For this review, take the finished solid that the model builds, in its own axes (mm). A direction names the side the tool comes from. Coordinates: 2 decimals unless noted, no trailing zeros. Order: outer loops, then holes, each group sorted by start corner. A loop starts at its lowest first (then second) coordinate and runs counter-clockwise, first axis right, second up. Notation, with made-up numbers: (35.5, 64.25) -> (74.5, 64.25) arc R26 ccw to (74.5, 83.25) -> close; hole circle Ø9 at (-32, -29.75). An arc over 180 degrees is marked (long way). Write item = value, one per line. Start each with the question number.
1) Draft analysis for pull direction Y (two halves, no side actions). For faces 5 (the face through (15.266, 67.285, 4.93)), 6 (the face through (0, 19, 0)), 7 (the face through (0, 10, 18)), state which applies: +Y half, -Y half, draft (parallel to the pull), parting line (faces both ways), or undercut.
2) Machinability: for faces 1 (the face through (-21, 41, 5)), 2 (the face through (22.4, 7.5, 18.2)), 3 (the face through (0, 0, 20)), 4 (the face through (0, 34, 10)), which of the approach directions +Z, -Z, +X, -X, +Y, -Y give a long, thin tool a straight path to every point of the face, cutting with its end or side? Answer none if there is none.
3) Insertion check: pin 1 Ø4.5 at (x, y) = (-8, -5.5) entering from +Z; pin 2 Ø3 at (y, z) = (58.5, 3) entering from -X; pin 3 Ø8 at (x, y) = (6.5, -4.5) entering from -Z; pin 4 Ø8 at (x, z) = (-20, 20) entering from +Y. Each pin has a flat end and moves straight along its axis. Give the tip position at first contact, or say it passes through.
4) Consider section B-B on x = -20. Give the boundary of the cut face in (y, z), and give its area (3 significant figures).
5) Consider section C-C on z = 6.5. Give the boundary of the cut face in (x, y).
6) Consider section A-A on y = 50. Give the boundary of the cut face in (x, z), and give its area (3 significant figures).
7) Consider section D-D on z = 12.5. Give the boundary of the cut face in (x, y).
8) Wall thickness on probe 1 along Y at (x, z) = (-15.5, 6); probe 2 along Y at (x, z) = (14, 5.75); probe 3 along Z at (x, y) = (-20, 6.65): over which ranges is each line inside the solid? List them lowest first. Write a range as [from, to].
from build123d import *

# Parameters (mm, degrees)
SKETCH_R        = 1.8
SKETCH_R_2      = 11.5
PAD_DEPTH       = 10
SKETCH001_W     = 60
SKETCH001_H     = 10
PAD001_DEPTH    = 20
SKETCH002_R     = 3
POCKET_DEPTH    = 5
SKETCH003_R     = 1.8
POCKET001_DEPTH = 5
SKETCH004_W     = 60
SKETCH004_H     = 10
PAD002_DEPTH    = 15
FILLET_R        = 6
FILLET001_R     = 2


with BuildPart() as part:
    # Sketch → Pad (new body)
    with BuildSketch(Plane.XY):
        Polygon((21, 10), (21, 70.493559), (-21, 70.493559), (-21, 10), (-30, 10), (-30, 0), (30, 0), (30, 10), align=None)
        with Locations((15.5, 34.5)):
            Circle(SKETCH_R, mode=Mode.SUBTRACT)
        with Locations((-15.5, 34.5)):
            Circle(SKETCH_R, mode=Mode.SUBTRACT)
        with Locations((0, 50)):
            Circle(SKETCH_R_2, mode=Mode.SUBTRACT)
        with Locations((15.5, 65.5)):
            Circle(SKETCH_R, mode=Mode.SUBTRACT)
        with Locations((-15.5, 65.5)):
            Circle(SKETCH_R, mode=Mode.SUBTRACT)
    extrude(amount=PAD_DEPTH)

    # Sketch001 (on Face15 of Pad) → Pad001 (join)
    with BuildSketch(Plane.XY.offset(10)):
        with Locations((0, 5)):
            Rectangle(SKETCH001_W, SKETCH001_H)
    extrude(amount=PAD001_DEPTH)

    # Sketch002 (on Face6 of Pad001) → Pocket (cut)
    with BuildSketch(Plane(origin=(0, 10, 0), x_dir=(-1, 0, 0), z_dir=(0, 1, 0))):
        with Locations((-20, 20)):
            Circle(SKETCH002_R)
        with Locations((20, 20)):
            Circle(SKETCH002_R)
    extrude(amount=-POCKET_DEPTH, mode=Mode.SUBTRACT)

    # Sketch003 (on Face23 of Pocket) → Pocket001 (cut)
    with BuildSketch(Plane(origin=(0, 5, 0), x_dir=(-1, 0, 0), z_dir=(0, 1, 0))):
        with Locations((-20, 20)):
            Circle(SKETCH003_R)
        with Locations((20, 20)):
            Circle(SKETCH003_R)
    extrude(amount=-POCKET001_DEPTH, mode=Mode.SUBTRACT)

    # Sketch004 (on Face11 of Pocket001) → Pad002 (join)
    with BuildSketch(Plane.XZ):
        with Locations((0, 5)):
            Rectangle(SKETCH004_W, SKETCH004_H)
    extrude(amount=PAD002_DEPTH)

    # Fillet
    fillet_edges = [part.edges().sort_by_distance(p)[0] for p in [
        (-21, 70.493559, 5),
        (21, 70.493559, 5),
        (-21, 10, 5),
        (21, 10, 5),
    ]]
    fillet(fillet_edges, radius=FILLET_R)

    # Fillet001
    fillet001_edges = [part.edges().sort_by_distance(p)[0] for p in [
        (30, 10, 20),
        (-30, 10, 20),
    ]]
    fillet(fillet001_edges, radius=FILLET001_R)


solid = part.part
Answer sheet:
q1.face_5 = undercut
q1.face_6 = draft
q1.face_7 = +Y half
q2.face_1 = +Z, -Z, -X, +Y
q2.face_2 = +Y
q2.face_3 = +Z, +X, -X, -Y
q2.face_4 = +Z, +X, -X, +Y
q3.pin_1 = 10
q3.pin_2 = -21
q3.pin_3 = 0
q3.pin_4 = 10
q4.outline = (-15, 0) -> (67.81, 0) -> (67.81, 10) -> (10, 10) -> (10, 17) -> (5, 17) -> (5, 18.2) -> (0, 18.2) -> (0, 10) -> (-15, 10) -> close; (0, 21.8) -> (5, 21.8) -> (5, 23) -> (10, 23) -> (10, 30) -> (0, 30) -> close
q4.area = 980 mm2
q5.outline = (-30, -15) -> (30, -15) -> (30, 8) arc R2 ccw to (28, 10) -> (27, 10) arc R6 cw to (21, 16) -> (21, 64.49) arc R6 ccw to (15, 70.49) -> (-15, 70.49) arc R6 ccw to (-21, 64.49) -> (-21, 16) arc R6 cw to (-27, 10) -> (-28, 10) arc R2 ccw to (-30, 8) -> close; hole circle Ø3.6 at (-15.5, 34.5); hole circle Ø3.6 at (-15.5, 65.5); hole circle Ø23 at (0, 50); hole circle Ø3.6 at (15.5, 34.5); hole circle Ø3.6 at (15.5, 65.5)
q6.outline = (-21, 0) -> (-11.5, 0) -> (-11.5, 10) -> (-21, 10) -> close; (11.5, 0) -> (21, 0) -> (21, 10) -> (11.5, 10) -> close
q6.area = 190 mm2
q7.outline = (-30, 0) -> (30, 0) -> (30, 8) arc R2 ccw to (28, 10) -> (-28, 10) arc R2 ccw to (-30, 8) -> close
q8.probe_1 = [-15, 32.7], [36.3, 63.7], [67.3, 70.47]
q8.probe_2 = [-15, 33.51], [35.49, 64.51], [66.49, 70.49]
q8.probe_3 = [0, 17], [23, 30]
